For this review, take the finished solid that the model builds, in its own axes (mm). Face numbers are marked on the shaded views. Give positions to 0.01 mm unless a question says otherwise; leave off trailing zeros. Order: outer loops, then holes, each group sorted by start corner. A loop starts at its lowest first (then second) coordinate and runs counter-clockwise, first axis right, second up. Notation, with made-up numbers: M 24,37 L 62,37 A9 cw 62,47 Z; hole C 81.5,-5 d7. An arc over 180 degrees is marked long. Use CSV: the item, a comma, the result in double quotes. Start each with the question number.
(1) Consider section A-A (y = 6.5). Write out the cut boundary in (x, z), and give its area (3 significant figures).
(2) Consider section B-B (z = -15). Write out the cut boundary in (x, y).
(3) Consider section D-D (z = -63.5). Write out the cut boundary in (x, y), and give its area (3 significant figures).
(4) Wall thickness on L1, parallel to Z at x = 0, y = 1.4; L2, parallel to X at y = 5.5, z = -49.5: over which ranges is each line inside the solid? List them lowest first. Write a range as from..to.
(5) Clearance check with flat-ended pins moving along their axes: P1, Ø5, axis at x = 0, z = 0, coming from the +Y side; P2, Ø4, axis at x = 25, y = 1, coming from the -Z side; P3, Ø1.1, axis at x = 33.5, y = 6, coming from the -Z side. State where each tip first meets the part, or that it passes through.
(6) Consider section C-C (x = -14). Write out the cut boundary in (y, z).
(7) Draft analysis for pull direction Z (two halves, no side actions). For the marked faces 1 and 2, state which applies: pulls with the +Z half, pulls with the -Z half, needs draft (parallel to the pull), parting line crosses it, or undercut.
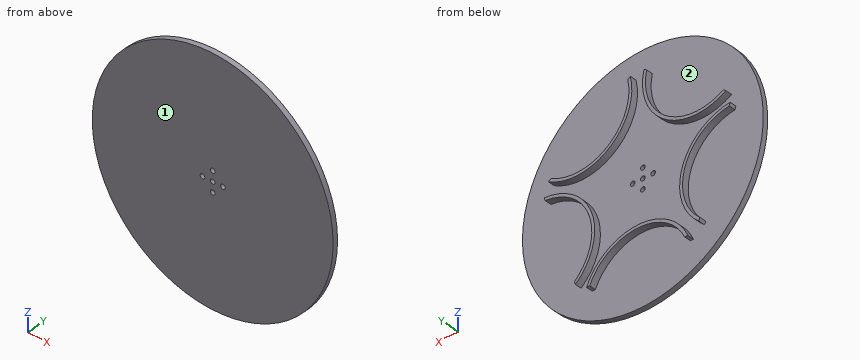
```python
from build123d import *

# Parameters (mm, degrees)
SKETCH_2_R      = 82.5
SKETCH_2_R_2    = 1.6
EXTRUDE_1_DEPTH = 3.5
EXTRUDE_2_DEPTH = 8


with BuildPart() as part:
    # Sketch 2 → Extrude 1 (new body)
    with BuildSketch(Plane(origin=(0, 0, 0), x_dir=(1, 0, 0), z_dir=(0, 1, 0))):
        Circle(SKETCH_2_R)
        Circle(SKETCH_2_R_2, mode=Mode.SUBTRACT)
        with Locations((0, 7)):
            Circle(SKETCH_2_R_2, mode=Mode.SUBTRACT)
        with Locations((7, 0)):
            Circle(SKETCH_2_R_2, mode=Mode.SUBTRACT)
        with Locations((0, -7)):
            Circle(SKETCH_2_R_2, mode=Mode.SUBTRACT)
        with Locations((-7, 0)):
            Circle(SKETCH_2_R_2, mode=Mode.SUBTRACT)
    extrude(amount=EXTRUDE_1_DEPTH)

    # Sketch 2_3 → Extrude 2 (add)
    with BuildSketch(Plane(origin=(0, 0, 0), x_dir=(1, 0, 0), z_dir=(0, 1, 0))):
        with BuildLine():
            ThreePointArc((59.042767356, -25.973094981), (20.278591204, -27.911086306), (6.456662722, -64.17913638))
            Line((6.456662722, -64.17913638), (4.698282977, -65.456674045))
            ThreePointArc((4.698282977, -65.456674045), (19.1030207, -26.293052317), (60.801147102, -24.695557316))
            Line((60.801147102, -24.695557316), (59.042767356, -25.973094981))
        make_face()
        with BuildLine():
            ThreePointArc((-63.033204373, -13.69179267), (-32.811449812, 10.661086306), (-42.947099738, 48.126880889))
            Line((-42.947099738, 48.126880889), (-42.275458441, 50.193980253))
            ThreePointArc((-42.275458441, 50.193980253), (-30.90933678, 10.043052317), (-63.70484567, -15.758892035))
            Line((-63.70484567, -15.758892035), (-63.033204373, -13.69179267))
        make_face()
        with BuildLine():
            ThreePointArc((-6.456662722, -64.17913638), (-20.278591204, -27.911086306), (-59.042767356, -25.973094981))
            Line((-59.042767356, -25.973094981), (-60.801147102, -24.695557316))
            ThreePointArc((-60.801147102, -24.695557316), (-19.1030207, -26.293052317), (-4.698282977, -65.456674045))
            Line((-4.698282977, -65.456674045), (-6.456662722, -64.17913638))
        make_face()
        with BuildLine():
            ThreePointArc((42.947099738, 48.126880889), (32.811449812, 10.661086306), (63.033204373, -13.69179267))
            Line((63.033204373, -13.69179267), (63.70484567, -15.758892035))
            ThreePointArc((63.70484567, -15.758892035), (30.90933678, 10.043052317), (42.275458441, 50.193980253))
            Line((42.275458441, 50.193980253), (42.947099738, 48.126880889))
        make_face()
        with BuildLine():
            ThreePointArc((-32.5, 55.717143143), (0, 34.5), (32.5, 55.717143143))
            Line((32.5, 55.717143143), (34.673476895, 55.717143143))
            ThreePointArc((34.673476895, 55.717143143), (0, 32.5), (-34.673476895, 55.717143143))
            Line((-34.673476895, 55.717143143), (-32.5, 55.717143143))
        make_face()
    extrude(amount=EXTRUDE_2_DEPTH)


solid = part.part
```
Check result:
1,outline,"M -63.7,15.76 L -63.03,13.69 A35.5 cw -42.95,-48.13 L -42.28,-50.19 A37.5 ccw Z; M -60.8,24.7 A37.5 ccw -4.7,65.46 L -6.46,64.18 A35.5 cw -59.04,25.97 Z; M -34.67,-55.72 L -32.5,-55.72 A35.5 cw 32.5,-55.72 L 34.67,-55.72 A37.5 ccw Z; M 4.7,65.46 A37.5 ccw 60.8,24.7 L 59.04,25.97 A35.5 cw 6.46,64.18 Z; M 42.28,-50.19 L 42.95,-48.13 A35.5 cw 63.03,13.69 L 63.7,15.76 A37.5 ccw Z"
1,area,"853 mm^2"
2,outline,"M -81.12,0 L 81.12,0 L 81.12,3.5 L 31.7,3.5 L 31.7,8 L 29.66,8 L 29.66,3.5 L -29.66,3.5 L -29.66,8 L -31.7,8 L -31.7,3.5 L -81.12,3.5 Z"
3,outline,"M -52.67,0 L 52.67,0 L 52.67,3.5 L -52.67,3.5 Z"
3,area,"369 mm^2"
4,L1,"z = -82.5..-8.6, -5.4..-1.6, 1.6..5.4, 8.6..82.5"
4,L2,"x = -42.5..-41.48, -31.4..-28.98, 28.98..31.4, 41.48..42.5"
5,P1,"stops at y = 3.5"
5,P2,"stops at z = -79.23"
5,P3,"stops at z = -55.72"
6,outline,"M 0,-81.3 L 3.5,-81.3 L 3.5,-37.38 L 8,-37.38 L 8,-35.21 L 3.5,-35.21 L 3.5,30.76 L 8,30.76 L 8,33.75 L 3.5,33.75 L 3.5,81.3 L 0,81.3 Z"
7,face 1,"needs draft"
7,face 2,"undercut"
